Read the model definition and answer for the solid it produces. Units are mm, in the model's axes. Face numbers are marked on the shaded views. A direction names the side the tool comes from. Give positions to 0.01 mm unless a question says otherwise; leave off trailing zeros. Loops run counter-clockwise (first coordinate to the right, second up) from the corner with the lowest first, then second, coordinate; pieces in that order, holes last. Notation, with made-up numbers: (89, 41) - (124, 41) arc R36 ccw to (124, 78) - close; hole circle Ø5 at (-22, -11). An arc over 180 degrees is marked (long way). Use a Markdown table: item, result. Add a question column.
Item 1: Each of these flat-tipped pins is pushed along its axis until it touches: P1, Ø4.5, axis at x = 20.5, z = 9, coming from the +Y side; P2, Ø3, axis at y = 4.5, z = 16.5, coming from the -X side; P3, Ø4, axis at x = -110.5, y = -2, coming from the +Z side; P4, Ø3, axis at x = -79, y = 12, coming from the +Z side. Where does it stop, or does it pass through?
Item 2: Which of the six approach directions +Z, -Z, +X, -X, +Y, -Y give full straight-line access (tool end or side, diameter ignored) to the marked faces 1 and 2?
Item 3: A cutting plane is placed at C-C (x = -80). Determine the outline of the cut face in (y, z), plus the area to 3 significant figures.
Item 4: For a pull along Y with two mould halves and no side action, classify the marked faces 3, 4, 5 and 6 as +Y half, -Y half, draft (parallel to the pull), parting line (faces both ways), or undercut.
Item 5: A cutting plane is placed at B-B (x = -19). Determine the outline of the cut face in (y, z), plus the area to 3 significant figures.
Item 6: A cutting plane is placed at D-D (z = 20). Determine the outline of the cut face in (x, y), plus the area to 3 significant figures.
Item 7: A cutting plane is placed at A-A (z = 7.5). Determine the outline of the cut face in (x, y), plus the area to 4 significant figures.
Item 8: Consider probe 1 along X at (y, z) = (-2.55, 7.5); probe 2 along Y at (x, z) = (-54, 25); probe 3 along X at (y, z) = (-3, 7). Determine where each line is inside the solid, lowest interval first. Write a range as [from, to].
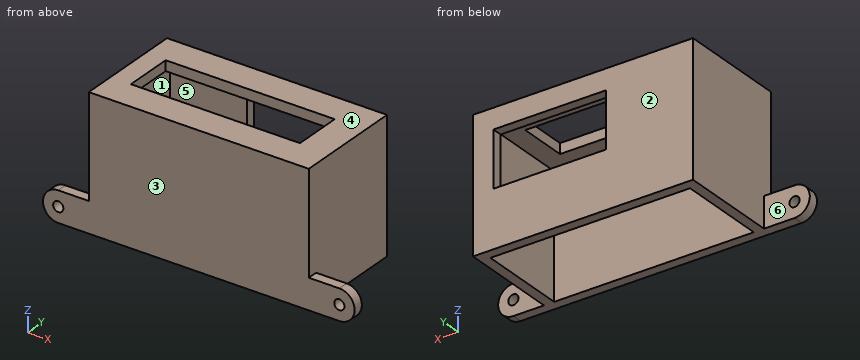
Autodesk Inventor part; units mm, degrees
ref_plane "YZ Plane" through (0, 0, 0) normal (1, 0, 0) x (0, 1, 0)
ref_plane "XZ Plane" through (0, 0, 0) normal (0, 1, 0) x (-1, 0, 0)
ref_plane "XY Plane" through (0, 0, 0) normal (0, 0, 1) x (1, 0, 0)
sketch "Sketch1" plane through (0, 0, 0) normal (0, 0, 1) x (1, 0, 0)
  line L0 (0, 0) -> (-98, 0)
  line L1 (-98, 0) -> (-98, 44)
  line L2 (-98, 44) -> (0, 44)
  line L3 (0, 44) -> (0, 0)
  line L4 (5, -5) -> (-103, -5)
  line L5 (-103, -5) -> (-103, 49)
  line L6 (-103, 49) -> (5, 49)
  line L7 (5, 49) -> (5, -5)
  dimension "d0" = 98
  dimension "d1" = 44
  dimension "d2" = 5
  dimension "d3" = 5
  dimension "d4" = 5
  dimension "d5" = 5
extrude "Extrusion1" add sketch "Sketch1" along normal blind 60
sketch "Sketch2" plane through (0, 0, 60) normal (0, 0, 1) x (1, 0, 0)
  line L0 (5, 49) -> (-103, 49)
  line L1 (5, -5) -> (-103, -5)
  line L2 (-103, -5) -> (-103, 49)
  line L3 (-103, 49) -> (5, 49)
  line L4 (5, 49) -> (5, -5)
  line L5 (-93, 34) -> (-10, 34)
  line L6 (-10, 34) -> (-10, 10)
  line L7 (-10, 10) -> (-93, 10)
  line L8 (-93, 10) -> (-93, 34)
  point P0 (0, 0)
  dimension "d10" = 10
  dimension "d11" = 15
  dimension "d12" = 15
  dimension "d13" = 15
extrude "Extrusion2" add sketch "Sketch2" along normal blind 5
sketch "Sketch4" plane through (-103, 49, 0) normal (0, 1, 0) x (1, 0, 0)
  line L0 (98, -27.8) -> (42.8, -27.8)
  line L1 (42.8, -27.8) -> (42.8, -55)
  line L2 (42.8, -55) -> (98, -55)
  line L3 (98, -55) -> (98, -27.8)
  line L4 (108, -65) -> (0, -65)
  line L5 (108, 0) -> (108, -65)
  point P0 (103, 0)
  dimension "d19" = 27.2
  dimension "d20" = 55.2
  dimension "d21" = 10
  dimension "d22" = 10
extrude "Extrusion4" cut sketch "Sketch4" against normal blind 10
sketch "Sketch5" plane through (-103, -5, 0) normal (0, -1, 0) x (1, 0, 0)
  line L0 (108, 0) -> (108, 65)
  line L1 (108, 0) -> (123, 0)
  line L2 (123, 0) -> (123, 15)
  line L3 (123, 15) -> (108, 15)
  line L4 (108, 15) -> (108, 0)
  circle A0 centre (123, 7.5) radius 7.5
  circle A1 centre (123, 7.5) radius 2.5
  line L5 (103, 0) -> (5, 0)
  line L6 (54, 0) -> (54, -10.2425)
  line L7 (0, 0) -> (-15, 0)
  line L8 (-15, 0) -> (-15, 15)
  line L9 (-15, 15) -> (0, 15)
  line L10 (0, 15) -> (0, 0)
  circle A2 centre (-15, 7.5) radius 7.5
  circle A3 centre (-15, 7.5) radius 2.5
  dimension "d25" = 15
  dimension "d26" = 5
  dimension "d27" = 15
extrude "Extrusion5" add sketch "Sketch5" against normal blind 5 contours L0 L3 A0 L1 | A0 L2 A1 | L2 A1 A0 | L7 A2 L9 L10 | A2 L8 A3 | L8 A3 A2
equation "\"d27\" = d25"
equation "\"RodDiameter\" = 8"
equation "\"VerticalBearingOD\" = 16"
equation "\"PrintingClearance\" = 0.2"
equation "\"TubeID\" = 18"
properties part number "PSUBracket"
Geometry says:
| question | item | result |
|---|---|---|
| 1 | P1 | y = 0 |
| 1 | P2 | x = -103 |
| 1 | P3 | z = 15 |
| 1 | P4 | through |
| 2 | face 1 | -Z |
| 2 | face 2 | +Z, -Z, +X, -X, +Y |
| 3 | outline | (-5, 0) - (0, 0) - (0, 60) - (10, 60) - (10, 65) - (-5, 65) - close; (34, 60) - (44, 60) - (44, 0) - (49, 0) - (49, 65) - (34, 65) - close |
| 3 | area | 750 mm² |
| 4 | face 3 | -Y half |
| 4 | face 4 | draft |
| 4 | face 5 | undercut |
| 4 | face 6 | +Y half |
| 5 | outline | (-5, 0) - (0, 0) - (0, 60) - (10, 60) - (10, 65) - (-5, 65) - close; (34, 60) - (44, 60) - (44, 55) - (49, 55) - (49, 65) - (34, 65) - close; (44, 0) - (49, 0) - (49, 27.8) - (44, 27.8) - close |
| 5 | area | 614 mm² |
| 6 | outline | (-103, -5) - (5, -5) - (5, 49) - (-103, 49) - close; hole (-98, 0) - (0, 0) - (0, 44) - (-98, 44) - close |
| 6 | area | 1,520 mm² |
| 7 | outline | (-125.5, -5) - (-120.5, -5) - (-120.5, 0) - (-125.5, 0) - close; (-115.5, -5) - (17.5, -5) - (17.5, 0) - (5, 0) - (5, 49) - (-103, 49) - (-103, 0) - (-115.5, 0) - close; (22.5, -5) - (27.5, -5) - (27.5, 0) - (22.5, 0) - close; hole (-98, 0) - (0, 0) - (0, 44) - (-98, 44) - close |
| 7 | area | 1,695 mm² |
| 8 | probe 1 | [-125.5, -120.5], [-115.5, 17.5], [22.5, 27.5] |
| 8 | probe 2 | [-5, 0], [44, 49] |
| 8 | probe 3 | [-125.48, -120.45], [-115.55, 17.55], [22.45, 27.48] |
